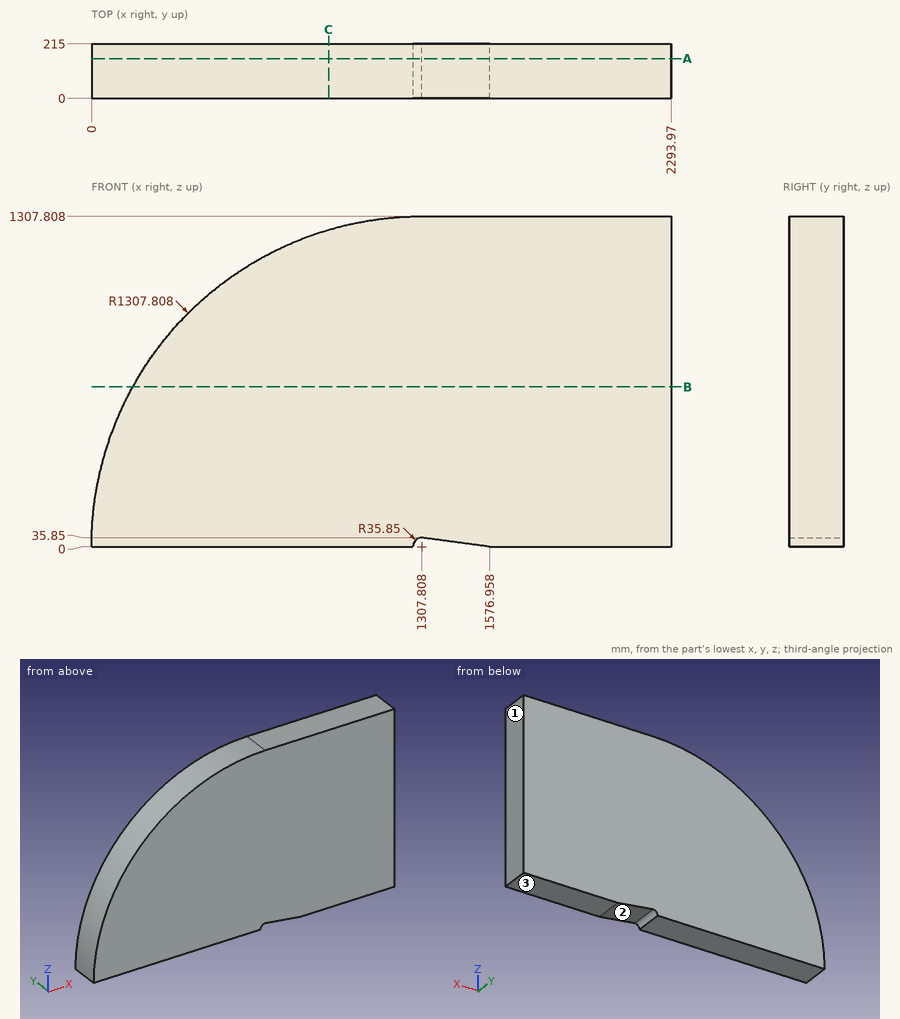
Here's the drawing with two shaded views (mm, measured from the low corner). I have some questions. Coordinates: 2 decimals unless noted, no trailing zeros. Write each loop counter-clockwise with the first axis right and the second up, starting at its lowest first coordinate (ties: lowest second). Pieces come first, ordered by that corner, then holes. Notation, with made-up numbers: (14.25, 87) -> (41.25, 87) arc R22 cw to (41.25, 117) -> close; hole circle Ø4 at (80, -6). An arc over 180 degrees is marked (long way). Use a Markdown table: item, result. Add a question column.
(1) Please list where these lines run through material, in increasing order: line 1 (X direction, y = 153, z = 480); line 2 (Z direction, x = 443, y = 86.5) (1 decimal); line 3 (Z direction, x = 130, y = 205.5) (1 decimal).
(2) If we section it at A-A, the plane y = 157.5: Write out the boundary of the cut face in (x, z), and give its area (3 significant figures).
(3) If we section it at C-C, the plane x = 938.5: Write out the boundary of the cut face in (y, z).
(4) If we section it at B-B, the plane z = 633: Write out the boundary of the cut face in (x, y).
(5) We'd pull the mould along X, two halves only. Please class the marked faces 1, 2 and 3: +X half, -X half, draft (parallel to the pull), parting line (faces both ways), or undercut.
(6) I'm going to push a flat-ended pin straight in: P1, Ø6, axis at y = 145.5, z = 941.5, coming from the -X side (1 decimal). Where does the tip first touch, or does it pass through?
Outcome:
| question | item | result |
|---|---|---|
| 1 | line 1 | x = 91.27 to 2293.97 |
| 1 | line 2 | z = 0 to 981.1 |
| 1 | line 3 | z = 0 to 568.4 |
| 2 | outline | (0, 0) -> (1271.96, 0) arc R35.85 cw to (1307.81, 35.85) -> (1576.96, 0) -> (2293.97, 0) -> (2293.97, 1307.81) -> (1307.81, 1307.81) arc R1307.81 ccw to start |
| 2 | area | 2,630,000 mm^2 |
| 3 | outline | (0, 0) -> (215, 0) -> (215, 1254.58) -> (0, 1254.58) -> close |
| 4 | outline | (163.4, 0) -> (2293.97, 0) -> (2293.97, 215) -> (163.4, 215) -> close |
| 5 | face 1 | +X half |
| 5 | face 2 | undercut |
| 5 | face 3 | draft |
| 6 | P1 | stops at x = 397 |
